The figure shows three views and two pictorial views of one solid part (mm, origin at its lowest corner). Answer the questions. A direction names the side the tool comes from. Round coordinates to 2 decimals unless told otherwise and drop trailing zeros. Order: outer loops, then holes, each group sorted by start corner. A loop starts at its lowest first (then second) coordinate and runs counter-clockwise, first axis right, second up.
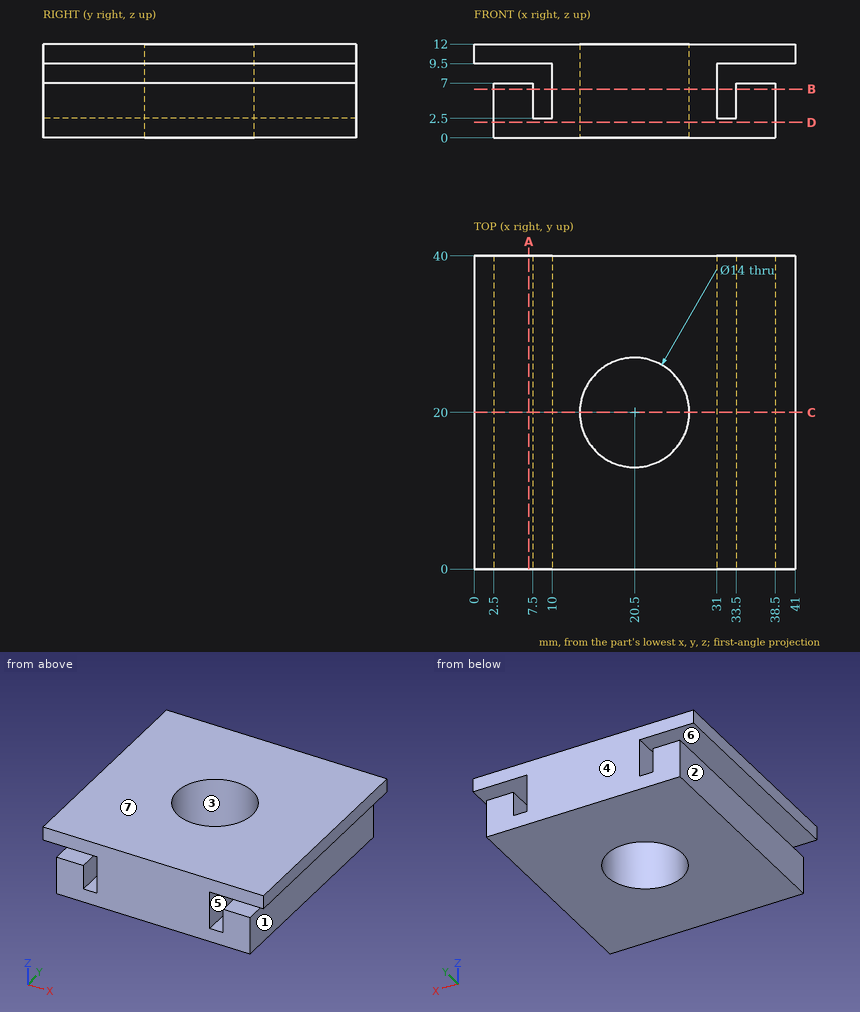
Item 1: A tool of negligible diameter and unlimited length cuts with its end or side. For the marked faces 5, 6 and 7, from which of +Z, -Z, +X, -X, +Y, -Y can it reach the whole face along a straight path? Write none if from no direction.
Item 2: Find section A-A (x = 7). Write down the section's boundary in (y, z).
Item 3: Find the intervals of material crossed by line 1 along X through (y, z) = (20, 6); line 2 along Z through (x, y) = (5.5, 7); line 3 along X through (y, z) = (20, 7.5), in increasing order.
Item 4: For a pull along X with two mould halves and no side action, classify the marked faces 1, 2, 3 and 4 as released by +X, released by -X, zero draft, split by the parting line, or undercut.
Item 5: Find section C-C (y = 20). Write down the section's boundary in (x, z), plus the area to 4 significant figures.
Item 6: Find section B-B (z = 6.25). Write down the section's boundary in (x, y), plus the area to 3 significant figures.
Item 7: Given pin 1 (2 mm diameter, centred on y = 12, z = 5.5, fed in from +X); pin 2 (2 mm diameter, centred on y = 16, z = 4, fed in from -X); pin 3 (6 mm diameter, centred on x = 20, y = 19, fed in from +Z), each flat-ended and moving along its own axis, determine where each tip first touches the part or whether it passes through.
Item 8: Find section D-D (z = 2). Write down the section's boundary in (x, y), plus the area to 3 significant figures.
Model answer:
1. face 5: +Y, -Y
1. face 6: -X, +Y, -Y
1. face 7: +Z, +X, -X, +Y, -Y
2. outline: (0, 0) - (40, 0) - (40, 7) - (0, 7) - close; (0, 9.5) - (40, 9.5) - (40, 12) - (0, 12) - close
3. line 1: x = 2.5 to 7.5, 10 to 13.5, 27.5 to 31, 33.5 to 38.5
3. line 2: z = 0 to 7, 9.5 to 12
3. line 3: x = 10 to 13.5, 27.5 to 31
4. face 1: released by +X
4. face 2: released by -X
4. face 3: undercut
4. face 4: zero draft
5. outline: (0, 9.5) - (10, 9.5) - (10, 2.5) - (7.5, 2.5) - (7.5, 7) - (2.5, 7) - (2.5, 0) - (13.5, 0) - (13.5, 12) - (0, 12) - close; (27.5, 0) - (38.5, 0) - (38.5, 7) - (33.5, 7) - (33.5, 2.5) - (31, 2.5) - (31, 9.5) - (41, 9.5) - (41, 12) - (27.5, 12) - close
5. area: 216.5 mm2
6. outline: (2.5, 0) - (7.5, 0) - (7.5, 40) - (2.5, 40) - close; (10, 0) - (31, 0) - (31, 40) - (10, 40) - close; (33.5, 0) - (38.5, 0) - (38.5, 40) - (33.5, 40) - close; hole circle Ø14 at (20.5, 20)
6. area: 1,090 mm2
7. pin 1: stops at x = 38.5
7. pin 2: stops at x = 2.5
7. pin 3: passes through
8. outline: (2.5, 0) - (38.5, 0) - (38.5, 40) - (2.5, 40) - close; hole circle Ø14 at (20.5, 20)
8. area: 1,290 mm2
